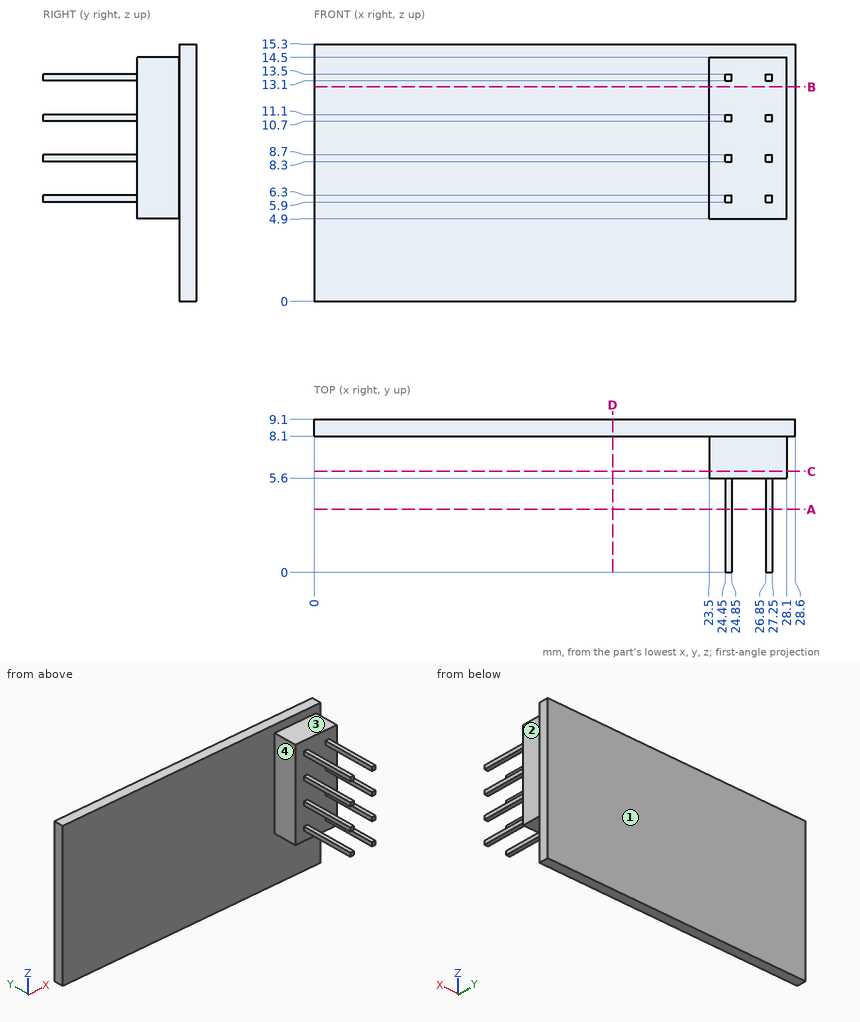
Here's the drawing with two shaded views (mm, measured from the low corner). I have some questions. A direction names the side the tool comes from. Give positions to 0.01 mm unless a question says otherwise; leave off trailing zeros. Loops run counter-clockwise (first coordinate to the right, second up) from the corner with the lowest first, then second, coordinate; pieces in that order, holes last. Notation, with made-up numbers: M 28,50 L 34,50 A22 ccw 34,71 Z; hole C 25,82 d6. An arc over 180 degrees is marked long. One line per item, written item: value.
(1) Which directions (+Z, -Z, +X, -X, +Y, -Y) give clear straight access to the entire face, cutting with the end or side of a thin tool? Please do the marked faces 1, 2, 3 and 4.
Returned:
face 1: +Z, -Z, +X, -X, +Y
face 2: +Z, -Z, +X, -Y
face 3: +Z, +X, -X, -Y
face 4: +Z, -Z, -X, -Y
(2) Suppose I cut it at C-C on y = 6. List the corners of the cut face in (x, z) for me, plus the area to 3 significant figures.
Returned:
outline: M 23.5,4.9 L 28.1,4.9 L 28.1,14.5 L 23.5,14.5 Z
area: 44.2 mm^2
(3) I need wall thicknesses on line 1 (Y direction, x = 3.75, z = 6.75); line 2 (X direction, y = 4.75, z = 13.25); line 3 (X direction, y = 6.25, z = 11.5). Which ranges of each line are inside material? Lowest first, please.
Returned:
line 1: 8.1 to 9.1
line 2: 24.45 to 24.85, 26.85 to 27.25
line 3: 23.5 to 28.1
(4) Will these pins go through, and if not, where does the flat tip stop? pin 1 (3 mm diameter, centred on y = 4, z = 3.5, fed in from +X); pin 2 (1 mm diameter, centred on x = 19, z = 11.5, fed in from -Y); pin 3 (4 mm diameter, centred on y = 1.5, z = 12.5, fed in from +X).
Returned:
pin 1: through
pin 2: y = 8.1
pin 3: x = 27.25
(5) Suppose I cut it at B-B on z = 12.75. List the corners of the cut face in (x, y) for me.
Returned:
outline: M 0,8.1 L 23.5,8.1 L 23.5,5.6 L 28.1,5.6 L 28.1,8.1 L 28.6,8.1 L 28.6,9.1 L 0,9.1 Z
(6) Suppose I cut it at D-D on x = 17.75. List the corners of the cut face in (y, z) for me.
Returned:
outline: M 8.1,0 L 9.1,0 L 9.1,15.3 L 8.1,15.3 Z
(7) Suppose I cut it at A-A on y = 3.75. Count the separate pieces of the cut face and the enclosed holes in it, plus the area to 3 significant figures.
Returned:
separate pieces: 8
enclosed holes: 0
area: 1.28 mm^2
